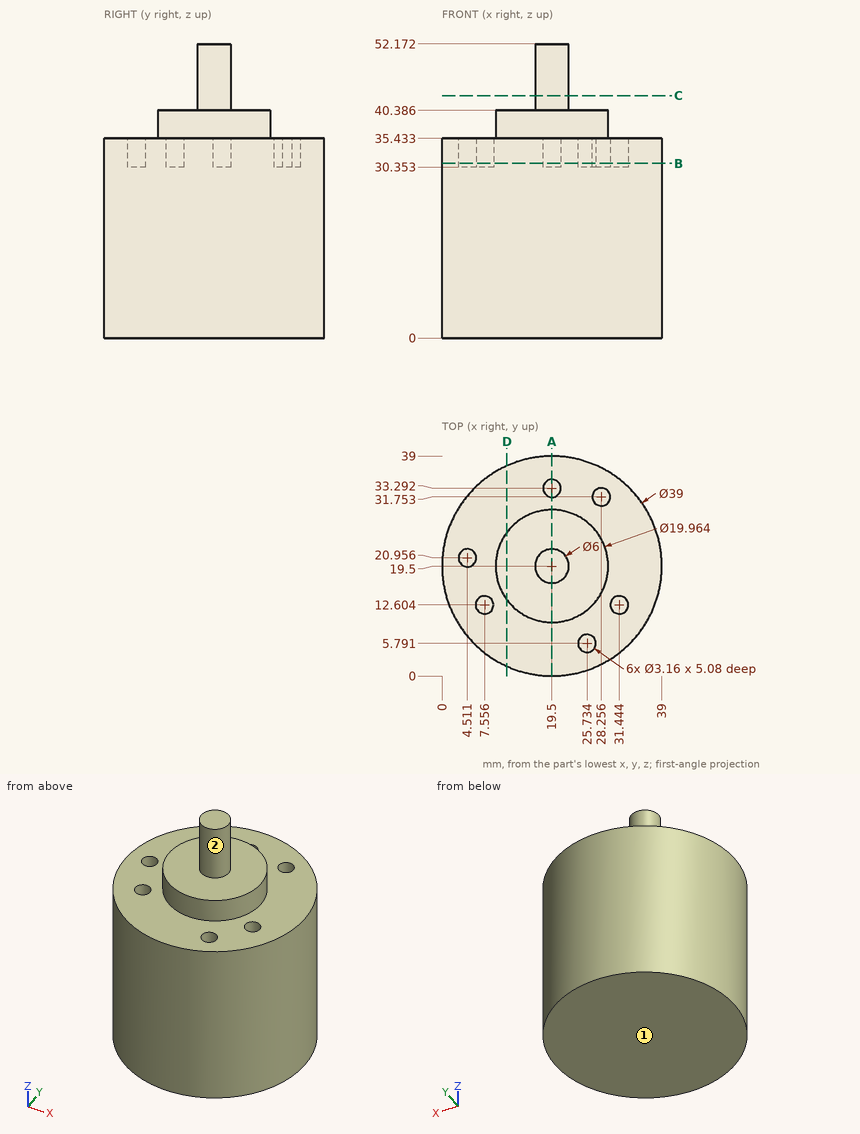
Study the drawing (mm; zero at the part's minimum x, y, z) and answer. A direction names the side the tool comes from. Round coordinates to 2 decimals unless told otherwise and drop trailing zeros. Loops run counter-clockwise (first coordinate to the right, second up) from the corner with the lowest first, then second, coordinate; pieces in that order, holes last. Notation, with made-up numbers: M 87,37.5 L 107,37.5 A19 ccw 107,52.5 Z; hole C 17.25,58 d8. An arc over 180 degrees is marked long. One line per question, with ' | ' between items.
Q1. Each of these flat-tipped pins is pushed along its axis until it touches: pin 1 Ø12 at (x, y) = (32.5, 9) entering from +Z; pin 2 Ø4 at (x, y) = (21.5, 26) entering from +Z; pin 3 Ø3 at (x, z) = (25.5, 33.5) entering from +Y. Where does it stop, or does it pass through?
Conclusion:
pin 1: stops at z = 35.43 | pin 2: stops at z = 40.39 | pin 3: stops at y = 38.47
Q2. Find section C-C, the plane z = 43. Give the vertices of the cut face in (x, y).
Conclusion:
outline: C 19.5,19.5 d6
Q3. A tool of negligible diameter and unlimited length cuts with its end or side. For the marked faces 1 and 2, from which of +Z, -Z, +X, -X, +Y, -Y can it reach the whole face along a straight path? Write none if from no direction.
Conclusion:
face 1: -Z, +X, -X, +Y, -Y | face 2: +Z
Q4. Consider line 1 along Z through (x, y) = (27.5, 26); line 2 along Y through (x, z) = (19.5, 9); line 3 along Y through (x, z) = (31.5, 29). Determine where each line is inside the solid, lowest interval first. Write a range as from..to.
Conclusion:
line 1: z = 0..35.43 | line 2: y = 0..39 | line 3: y = 4.13..34.87
Q5. Find section B-B, the plane z = 31. Give the vertices of the cut face in (x, y) (1 decimal).
Conclusion:
outline: C 19.5,19.5 d39; hole C 4.5,21 d3.2; hole C 7.6,12.6 d3.2; hole C 19.5,33.3 d3.2; hole C 25.7,5.8 d3.2; hole C 28.3,31.8 d3.2; hole C 31.4,12.6 d3.2
Q6. Find section D-D, the plane x = 11.5. Give the vertices of the cut face in (y, z).
Conclusion:
outline: M 1.72,0 L 37.28,0 L 37.28,35.43 L 25.47,35.43 L 25.47,40.39 L 13.53,40.39 L 13.53,35.43 L 1.72,35.43 Z
Q7. Find section A-A, the plane x = 19.5. Give the vertices of the cut face in (y, z), then the cut area to 3 significant figures.
Conclusion:
outline: M 0,0 L 39,0 L 39,35.43 L 34.87,35.43 L 34.87,30.35 L 31.71,30.35 L 31.71,35.43 L 29.48,35.43 L 29.48,40.39 L 22.5,40.39 L 22.5,52.17 L 16.5,52.17 L 16.5,40.39 L 9.52,40.39 L 9.52,35.43 L 0,35.43 Z | area: 1,540 mm2
